Verification items for the finished model (mm, model axes). A direction names the side the tool comes from. Coordinates: 2 decimals unless noted, no trailing zeros. Write each loop counter-clockwise with the first axis right and the second up, starting at its lowest first coordinate (ties: lowest second). Pieces come first, ordered by that corner, then holes. Notation, with made-up numbers: (43.5, 73.25) -> (69.5, 73.25) arc R19 cw to (69.5, 102.25) -> close; hole circle Ø3 at (-36.75, 47.25). An arc over 180 degrees is marked (long way). Write item = value, one per line. Start each with the question number.
(1) Section check D-D (x = 69). Record the cut outline in (y, z).
(2) Section check B-B (y = -17.5). Record the cut outline in (x, z).
(3) Section check C-C (x = 43). Record the cut outline in (y, z), plus the area to 3 significant figures.
(4) Material ranges on probe 1 along Y at (x, z) = (89.5, -4); probe 2 along X at (y, z) = (-90.5, -2.25); probe 3 along Z at (x, y) = (2.95, -48), recorded low to high. Write a range as [from, to].
(5) Gauge pin test, flat ends, axial feed: pin 1 Ø4 at (x, z) = (88, -3.5) entering from +Y; pin 2 Ø5 at (x, y) = (22, -84.5) entering from -Z; pin 3 Ø1.5 at (y, z) = (-46.5, -3.5) entering from -X; pin 4 Ø1.2 at (y, z) = (-93, -4) entering from -X. Record the tip position at first contact, or that the pin passes through.
(6) Mould release check, pull along X, two halves, no side actions. Record for faces 1 (the face through (5, -90, -4)), 2 (the face through (2, -43, -4)): released by +X, released by -X, zero draft, split by the parting line, or undercut.
(7) Set-up check for faces 3 (the face through (89, -43, -4)), 4 (the face through (45, -93, -3)), 5 (the face through (76, -96, -4)), 6 (the face through (2, -88, -4)), 7 (the face through (45, -47, 2)): record each of +Z, -Z, +X, -X, +Y, -Y from which the full face is reachable in a straight line by a thin tool's end or side.
(8) Section check A-A (y = -4). Record the cut outline in (x, z).
Autodesk Inventor part; units mm, degrees
ref_plane "YZ Plane" through (0, 0, 0) normal (1, 0, 0) x (0, 1, 0)
ref_plane "XZ Plane" through (0, 0, 0) normal (0, 1, 0) x (-1, 0, 0)
ref_plane "XY Plane" through (0, 0, 0) normal (0, 0, 1) x (1, 0, 0)
ref_plane "Work Plane1" through (0, 0, 0) normal (0, 0, 1) x (1, 0, 0)
sketch "Sketch1" plane through (0, 0, 0) normal (0, 0, 1) x (1, 0, 0)
  line L0 (0, 2) -> (91, 2)
  line L1 (51.2, -11.9194) -> (39.8, -11.9194)
  line L2 (39.5, -11.9194) -> (39.5, -22.3444)
  line L3 (40.05, -22.8694) -> (50.95, -22.8694)
  line L4 (51.5, -11.9194) -> (51.5, -22.3444)
  line L5 (39.5, -11.9194) -> (51.5, -11.9194)
  line L6 (51.5, -11.9194) -> (51.5, -22.8694)
  line L7 (51.5, -22.8694) -> (39.5, -22.8694)
  line L8 (39.5, -22.8694) -> (39.5, -11.9194)
  line L9 (0, 2) -> (91, 2)
  line L10 (91, 2) -> (91, -98)
  line L11 (91, -98) -> (0, -98)
  line L12 (0, -98) -> (0, 2)
  circle A0 centre (5, -4) radius 0.75
  circle A1 centre (43, -4) radius 0.75
  circle A2 centre (81, -4) radius 0.75
  circle A3 centre (5, -4) radius 1.75
  circle A4 centre (43, -4) radius 1.75
  circle A5 centre (81, -4) radius 1.75
  point P0 (0, 0)
  dimension "d0" = 91
  dimension "d1" = 100
  dimension "d2" = 1
  dimension "d3" = 1
  dimension "d4" = 1
extrude "Extrusion1" add sketch "Sketch1" along normal blind 2 contours L0 L10 L11 L12
sketch "Sketch2" plane through (0, 0, 0) normal (0, 0, -1) x (-1, 0, 0)
  line L0 (-91, 2) -> (0, 2)
  line L1 (0, 2) -> (-91, 2)
  point P0 (0, 0)
sketch "Sketch3" plane through (0, 0, 0) normal (0, 0, -1) x (-1, 0, 0)
  point P0 (0, 0)
sketch "Sketch4" plane through (0, -98, 0) normal (-1, 0, 0) x (0, 0, 1)
  line L0 (0, 100) -> (0, 0)
  circle A0 centre (-4, 50) radius 0.75
  line L1 (-8, 50) -> (-8, 55)
  line L2 (-8, 55) -> (0, 55)
  line L3 (0, 55) -> (0, 45)
  line L4 (0, 45) -> (-8, 45)
  line L5 (-8, 45) -> (-8, 50)
  point P0 (0, 98)
  dimension "d8" = 1.5
  dimension "d9" = 4
  dimension "d10" = 5
  dimension "d11" = 8
  dimension "d12" = 10
  dimension "d13" = 8
extrude "Extrusion2" add sketch "Sketch4" against normal blind 5
sketch "Sketch5" plane through (0, -98, 2) normal (-1, 0, 0) x (0, 0, 1)
  line L0 (-2, 0) -> (-2, 45)
  line L1 (-2, 0) -> (-10, 0)
  line L2 (-10, 0) -> (-10, 10)
  line L3 (-10, 10) -> (-2, 10)
  line L4 (-2, 10) -> (-2, 0)
  circle A0 centre (-6, 5) radius 0.75
  point P0 (-2, 98)
  dimension "d16" = 8
  dimension "d17" = 10
  dimension "d19" = 1.5
extrude "Extrusion3" add sketch "Sketch5" against normal blind 5
sketch "Sketch6" plane through (0, -98, 2) normal (0, -1, 0) x (1, 0, 0)
  line L0 (5, -10) -> (5, -2)
  line L1 (5, -2) -> (15, -2)
  line L2 (15, -2) -> (15, -10)
  line L3 (15, -10) -> (5, -10)
  line L4 (5, -10) -> (5, -2)
  circle A0 centre (10, -6) radius 0.75
  point P0 (0, -2)
  dimension "d22" = 10
  dimension "d23" = 8
  dimension "d25" = 1.5
extrude "Extrusion4" add sketch "Sketch6" against normal blind 5
sketch "Sketch7" plane through (91, -98, 0) normal (1, 0, 0) x (0, 0, -1)
  circle A0 centre (4, 50) radius 0.75
  circle A1 centre (4, 50) radius 0.75
  line L0 (8, 45) -> (0, 45)
  line L1 (0, 55) -> (8, 55)
  line L2 (0, 45) -> (8, 45)
  line L3 (8, 45) -> (8, 55)
  line L4 (8, 55) -> (0, 55)
  line L5 (0, 55) -> (0, 45)
  point P0 (0, 98)
extrude "Extrusion5" add sketch "Sketch7" against normal blind 5
sketch "Sketch8" plane through (91, -98, 2) normal (1, 0, 0) x (0, 0, -1)
  arc A0 (6.75, 5) -> (5.25, 5) centre (6, 5) ccw
  circle A1 centre (6, 5) radius 0.75
  line L0 (10, 10) -> (2, 10)
  line L1 (2, 0) -> (10, 0)
  line L2 (10, 10) -> (2, 10)
  line L3 (2, 10) -> (2, 0)
  line L4 (2, 0) -> (10, 0)
  line L5 (10, 0) -> (10, 10)
  point P0 (2, 98)
extrude "Extrusion6" add sketch "Sketch8" against normal blind 5
sketch "Sketch9" plane through (0, -98, 2) normal (0, -1, 0) x (1, 0, 0)
  point P0 (0, -2)
sketch "Sketch10" plane through (0, -98, 2) normal (0, -1, 0) x (1, 0, 0)
  line L0 (86, -2) -> (15, -2)
  line L1 (86, -2) -> (76, -2)
  line L2 (76, -2) -> (76, -10)
  line L3 (76, -10) -> (86, -10)
  line L4 (86, -10) -> (86, -2)
  circle A0 centre (81, -6) radius 0.75
  point P0 (0, -2)
  dimension "d32" = 10
  dimension "d33" = 8
  dimension "d35" = 1.5
extrude "Extrusion7" add sketch "Sketch10" against normal blind 5
sketch "Sketch11" plane through (0, -98, 2) normal (0, -1, 0) x (1, 0, 0)
  line L0 (39.5, -2) -> (51.5, -2)
  circle A0 centre (45.5, -6) radius 0.75
  line L1 (45.5, -6) -> (45.5, -10)
  line L2 (45.5, -10) -> (40.5, -10)
  line L3 (40.5, -10) -> (40.5, -2)
  line L4 (40.5, -2) -> (50.5, -2)
  line L5 (50.5, -2) -> (50.5, -10)
  line L6 (50.5, -10) -> (45.5, -10)
  point P0 (0, -2)
  dimension "d39" = 1.5
  dimension "d40" = 4
  dimension "d41" = 5
  dimension "d42" = 8
  dimension "d43" = 10
  dimension "d44" = 8
extrude "Extrusion8" add sketch "Sketch11" against normal blind 5
properties part number "Before" material "Nylon 6/6"
Response:
q1.outline = (-98, 0) -> (2, 0) -> (2, 2) -> (-98, 2) -> close
q2.outline = (0, 0) -> (39.5, 0) -> (39.5, 2) -> (0, 2) -> close; (51.5, 0) -> (91, 0) -> (91, 2) -> (51.5, 2) -> close
q3.outline = (-98, -8) -> (-93, -8) -> (-93, 0) -> (-22.87, 0) -> (-22.87, 2) -> (-98, 2) -> close; (-11.92, 0) -> (-5.75, 0) -> (-5.75, 2) -> (-11.92, 2) -> close; (-2.25, 0) -> (2, 0) -> (2, 2) -> (-2.25, 2) -> close
q3.area = 211 mm2
q4.probe_1 = [-98, -93.75], [-92.25, -88], [-53, -48.75], [-47.25, -43]
q4.probe_2 = [0, 5], [86, 91]
q4.probe_3 = [-8, -4.75], [-3.25, 2]
q5.pin_1 = -43
q5.pin_2 = 0
q5.pin_3 = 0
q5.pin_4 = 5
q6.face_1 = undercut
q6.face_2 = zero draft
q7.face_3 = -Z, +X, -X, +Y
q7.face_4 = -Z, +Y
q7.face_5 = -Z, +Y, -Y
q7.face_6 = -Z, +X, -X
q7.face_7 = +Z, +X, -X, +Y, -Y
q8.outline = (0, 0) -> (3.25, 0) -> (3.25, 2) -> (0, 2) -> close; (6.75, 0) -> (41.25, 0) -> (41.25, 2) -> (6.75, 2) -> close; (44.75, 0) -> (79.25, 0) -> (79.25, 2) -> (44.75, 2) -> close; (82.75, 0) -> (91, 0) -> (91, 2) -> (82.75, 2) -> close
